Work out the finished part from the listing and answer in its coordinate system (mm). Coordinates: 2 decimals unless noted, no trailing zeros. Order: outer loops, then holes, each group sorted by start corner. A loop starts at its lowest first (then second) coordinate and runs counter-clockwise, first axis right, second up.
1. A flat-ended cylindrical pin translates along its axis: pin 1 Ø1 at (x, z) = (9.5, 4.5) entering from -Y. Find the tip coordinate at first contact, or state that the pin passes through.
2. Find the intervals of material crossed by probe 1 along X at (y, z) = (8.25, 5.75); probe 2 along X at (y, z) = (5, 4.75); probe 3 along X at (y, z) = (5, 2.5), in increasing order.
3. The part is cut by section B-B, the plane z = 4.5. Give the vertices of the cut face in (x, y).
4. The part is cut by section A-A, the plane x = 13.75. Give the vertices of the cut face in (y, z).
5. The part is cut by section D-D, the plane z = 1. Give the vertices of the cut face in (x, y).
6. The part is cut by section C-C, the plane y = 2.25. Give the vertices of the cut face in (x, z).
7. Determine the mould class of faces 1 (the flat face through (18.8, 5, 4)), 2 (the flat face through (9, 10.5, 5)), 3 (the cylindrical face through (4.72, 5.18, 7.44)) for opening direction X: +X half, -X half, draft (parallel to the pull), parting line (faces both ways), or undercut.
```python
from build123d import *

# Parameters (mm, degrees)
EXTRUDE_1_DEPTH   = 10.5
FILLET_1_R        = 1
HOLE_WIZARD_M31_D = 3.4


with BuildPart() as part:
    # Эскиз1 → Бобышка-Вытянуть1 (new body)
    with BuildSketch(Plane(origin=(0, 0, 0), x_dir=(1, 0, 0), z_dir=(0, 1, 0))):
        with BuildLine():
            Line((0, 0), (0, -8))
            Line((0, -8), (18.8, -8))
            Line((18.8, -8), (18.8, 0))
            ThreePointArc((18.8, 0), (9.4, -3.835773145), (0, 0))
        make_face()
    extrude(amount=EXTRUDE_1_DEPTH)

    # Скругление1
    fillet_1_edges = [part.edges().sort_by_distance(p)[0] for p in [
        (18.8, 5.25, 8),
        (0, 5.25, 8),
    ]]
    fillet(fillet_1_edges, radius=FILLET_1_R)

    # Отверстие с зазором M31 (through all)
    with Locations(Plane(origin=(0, 10.5, 0), x_dir=(1, 0, 0), z_dir=(0, 1, 0))):
        with Locations((4.350247301, -5.779226371), (14.350247301, -5.779226371)):
            Hole(HOLE_WIZARD_M31_D / 2)


solid = part.part
```
Geometry says:
1. pin 1: stops at y = 0
2. probe 1: x = 0 to 2.65, 6.05 to 12.65, 16.05 to 18.8
2. probe 2: x = 0 to 3, 5.7 to 13, 15.7 to 18.8
2. probe 3: x = 0 to 3.56, 15.24 to 18.8
3. outline: (0, 0) - (3.23, 0) - (3.23, 10.5) - (0, 10.5) - close; (5.47, 0) - (13.23, 0) - (13.23, 10.5) - (5.47, 10.5) - close; (15.47, 0) - (18.8, 0) - (18.8, 10.5) - (15.47, 10.5) - close
4. outline: (0, 3.11) - (10.5, 3.11) - (10.5, 4.19) - (0, 4.19) - close; (0, 7.37) - (10.5, 7.37) - (10.5, 8) - (0, 8) - close
5. outline: (0, 0) - (1.14, 0) - (1.14, 10.5) - (0, 10.5) - close; (17.66, 0) - (18.8, 0) - (18.8, 10.5) - (17.66, 10.5) - close
6. outline: (0, 0) arc R13.44 cw to (18.8, 0) - (18.8, 7) arc R1 ccw to (17.8, 8) - (1, 8) arc R1 ccw to (0, 7) - close; hole circle Ø3.4 at (4.35, 5.78); hole circle Ø3.4 at (14.35, 5.78)
7. face 1: +X half
7. face 2: draft
7. face 3: undercut
